Design review of the part built by this model. Coordinates are the model's own, in mm. Face numbers are marked on the shaded views. A direction names the side the tool comes from. Give positions to 0.01 mm unless a question says otherwise; leave off trailing zeros. Loops run counter-clockwise (first coordinate to the right, second up) from the corner with the lowest first, then second, coordinate; pieces in that order, holes last.
from build123d import *

# Parameters (mm, degrees)
SKETCH1_R           = 28.4
SKETCH1_R_2         = 2.6
SKETCH1_R_3         = 4
BOSS_EXTRUDE1_DEPTH = 6
SKETCH2_R           = 12
SKETCH2_R_2         = 4
BOSS_EXTRUDE2_DEPTH = 20.4


with BuildPart() as part:
    # Sketch1 → Boss-Extrude1 (new body)
    with BuildSketch(Plane.XY):
        Circle(SKETCH1_R)
        with Locations((0, 23.75)):
            Circle(SKETCH1_R_2, mode=Mode.SUBTRACT)
        with Locations((20.56810334, 11.875)):
            Circle(SKETCH1_R_2, mode=Mode.SUBTRACT)
        with Locations((20.56810334, -11.875)):
            Circle(SKETCH1_R_2, mode=Mode.SUBTRACT)
        with Locations((0, -23.75)):
            Circle(SKETCH1_R_2, mode=Mode.SUBTRACT)
        with Locations((-20.56810334, -11.875)):
            Circle(SKETCH1_R_2, mode=Mode.SUBTRACT)
        with Locations((-20.56810334, 11.875)):
            Circle(SKETCH1_R_2, mode=Mode.SUBTRACT)
        Circle(SKETCH1_R_3, mode=Mode.SUBTRACT)
    extrude(amount=BOSS_EXTRUDE1_DEPTH)

    # Sketch2 → Boss-Extrude2 (add)
    with BuildSketch(Plane.XY.offset(6)):
        Circle(SKETCH2_R)
        Circle(SKETCH2_R_2, mode=Mode.SUBTRACT)
    extrude(amount=BOSS_EXTRUDE2_DEPTH)


solid = part.part
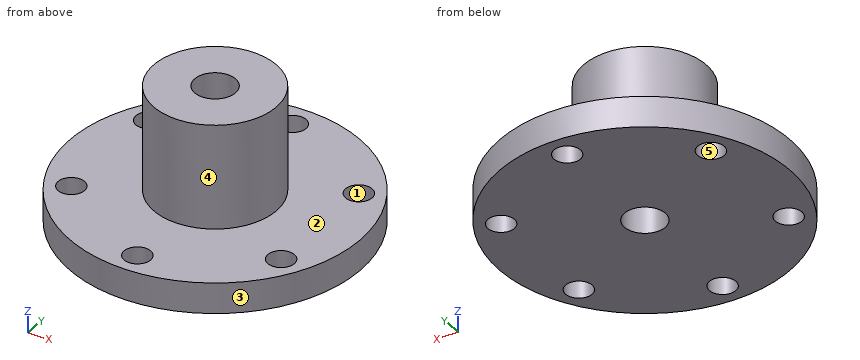
Q1. Tool access review of the marked faces 4 and 5: name each direction out of +Z, -Z, +X, -X, +Y, -Y from which nothing blocks a thin tool from reaching the whole face with its end or side.
Results:
face 4: +Z
face 5: +Z, -Z
Q2. Take a section at C-C (z = 22.75). Give the boundary of the cut face in (x, y).
Results:
outline: circle Ø24 at (0, 0); hole circle Ø8 at (0, 0)
Q3. Take a section at B-B (y = -23.75). Give the boundary of the cut face in (x, z), plus the area to 3 significant figures.
Results:
outline: (-15.57, 0) - (-2.6, 0) - (-2.6, 6) - (-15.57, 6) - close; (2.6, 0) - (15.57, 0) - (15.57, 6) - (2.6, 6) - close
area: 156 mm2
Q4. Take a section at D-D (x = -19.5). Give the boundary of the cut face in (y, z).
Results:
outline: (-20.65, 0) - (-14.25, 0) - (-14.25, 6) - (-20.65, 6) - close; (-9.5, 0) - (9.5, 0) - (9.5, 6) - (-9.5, 6) - close; (14.25, 0) - (20.65, 0) - (20.65, 6) - (14.25, 6) - close
Q5. Draft analysis for pull direction Y (two halves, no side actions). For the marked faces 1, 2 and 3, state which applies: pulls with the +Y half, pulls with the -Y half, needs draft (parallel to the pull), parting line crosses it, or undercut.
Results:
face 1: undercut
face 2: needs draft
face 3: parting line crosses it
Q6. Wall thickness on line 1 (Y direction, x = 0, z = 2.45); line 2 (Y direction, x = 0, z = 18.75); line 3 (Z direction, x = 22, y = 4): over which ranges is each line inside the solid? List them lowest first.
Results:
line 1: y = -28.4 to -26.35, -21.15 to -4, 4 to 21.15, 26.35 to 28.4
line 2: y = -12 to -4, 4 to 12
line 3: z = 0 to 6
Q7. Insertion check: pin 1 (2 mm diameter, centred on x = -15.5, y = 11, fed in from -Z); pin 2 (3 mm diameter, centred on x = -5.5, y = 13, fed in from +Z); pin 3 (6 mm diameter, centred on y = 0, z = 21, fed in from +X); pin 4 (6 mm diameter, centred on x = 5, z = 13.5, fed in from -Y). Each pin has a flat end and moves straight along its axis. Give the tip position at first contact, or say it passes through.
Results:
pin 1: stops at z = 0
pin 2: stops at z = 6
pin 3: stops at x = 12
pin 4: stops at y = -11.83
Q8. Take a section at A-A (x = 0). Give the boundary of the cut face in (y, z), plus the area to 3 significant figures.
Results:
outline: (-28.4, 0) - (-26.35, 0) - (-26.35, 6) - (-28.4, 6) - close; (-21.15, 0) - (-4, 0) - (-4, 26.4) - (-12, 26.4) - (-12, 6) - (-21.15, 6) - close; (4, 0) - (21.15, 0) - (21.15, 6) - (12, 6) - (12, 26.4) - (4, 26.4) - close; (26.35, 0) - (28.4, 0) - (28.4, 6) - (26.35, 6) - close
area: 557 mm2
